```python
from build123d import *

# Parameters (mm, degrees)
F0_W     = 500
F0_H     = 340
F0_W_2   = 280
F0_W_3   = 150
F0_H_2   = 30
F1_DEPTH = 400


with BuildPart() as f1:
    # F0 (on Front) → F1 (new body)
    with BuildSketch(Plane.XZ):
        Polygon((698.162909, 183.718975), (-701.837091, 183.718975), (-701.837091, 143.844262), (-701.837091, 143.718975), (-701.837091, -216.281025), (-551.837091, -216.281025), (548.162909, -216.281025), (698.162909, -216.281025), (698.162909, -186.281025), (698.162909, 153.718975), align=None)
        with Locations((-421.837091, -16.281025)):
            Rectangle(F0_W, F0_H, mode=Mode.SUBTRACT)
        with Locations((-1.837091, -16.281025)):
            Rectangle(F0_W_2, F0_H, mode=Mode.SUBTRACT)
        with Locations((418.162909, -16.281025)):
            Rectangle(F0_W, F0_H, mode=Mode.SUBTRACT)
        with Locations((623.162909, -231.281025)):
            Rectangle(F0_W_3, F0_H_2)
        with Locations((418.162909, -16.281025)):
            Rectangle(F0_W, F0_H)
        with Locations((-626.837091, -231.281025)):
            Rectangle(F0_W_3, F0_H_2)
    extrude(amount=F1_DEPTH)


solid = f1.part
```
Model file for the job. Use its own axes, mm. A direction names the side the tool comes from. Give positions to 0.01 mm unless a question says otherwise; leave off trailing zeros. Loops run counter-clockwise (first coordinate to the right, second up) from the corner with the lowest first, then second, coordinate; pieces in that order, holes last. Notation, with made-up numbers: (61.5, 0.25) - (109.5, 0.25) arc R13 cw to (109.5, 21.25) - close; hole circle Ø4 at (-32.5, -26). An arc over 180 degrees is marked (long way). One line per item, written item: value. Start each with the question number.
1. Probe L1, parallel to X at y = -207, z = -79.5; L2, parallel to Z at x = 69, y = -340; L3, parallel to Z at x = 513, y = -81. List the from-to ranges inside material, lowest first. Write a range as from..to.
2. Slice it at D-D (x = 307). List the corners of the cut face in (y, z).
3. Pin check, flat tip, straight feed: pin 1 (6 mm diameter, centred on x = -35, y = -224.5, fed in from -Z). Stop position of the tip, or through.
4. Which spindle directions (+Z, -Z, +X, -X, +Y, -Y) get a long thin tool onto all of the face, cutting with end or side? Do faces 1 (the flat face through (-141.837, -197, -19)), 2 (the flat face through (144, 0, 20)), 3 (the flat face through (548.163, -197, -231)). Say none if no direction does.
5. Pull direction Z, two halves, no side cores. Call faces 4 (the flat face through (8, -197, 183.719)), 5 (the flat face through (-10, -197, -216.281)), 6 (the flat face through (-671.837, -197, -19)): pulls with the +Z half, pulls with the -Z half, needs draft (parallel to the pull), parting line crosses it, or undercut.
6. Slice it at C-C (y = -167). List the corners of the cut face in (x, z), plus the area to 3 significant figures.
7. Slice it at B-B (z = -47.5). List the corners of the cut face in (x, y).
8. Slice it at A-A (x = -477.5). List the corners of the cut face in (y, z), plus the area to 3 significant figures.
Solution:
1. L1: x = -701.84..-671.84, -171.84..-141.84, 138.16..698.16
1. L2: z = -216.28..-186.28, 153.72..183.72
1. L3: z = -216.28..183.72
2. outline: (-400, -216.28) - (0, -216.28) - (0, 183.72) - (-400, 183.72) - close
3. pin 1: stops at z = -216.28
4. face 1: +Y, -Y
4. face 2: +Z, -Z, +X, -X, +Y
4. face 3: -Z, +Y, -Y
5. face 4: pulls with the +Z half
5. face 5: pulls with the -Z half
5. face 6: undercut
6. outline: (-701.84, -246.28) - (-551.84, -246.28) - (-551.84, -216.28) - (548.16, -216.28) - (548.16, -246.28) - (698.16, -246.28) - (698.16, 183.72) - (-701.84, 183.72) - close; hole (-671.84, -186.28) - (-171.84, -186.28) - (-171.84, 153.72) - (-671.84, 153.72) - close; hole (-141.84, -186.28) - (138.16, -186.28) - (138.16, 153.72) - (-141.84, 153.72) - close
6. area: 304,000 mm^2
7. outline: (-701.84, -400) - (-671.84, -400) - (-671.84, 0) - (-701.84, 0) - close; (-171.84, -400) - (-141.84, -400) - (-141.84, 0) - (-171.84, 0) - close; (138.16, -400) - (698.16, -400) - (698.16, 0) - (138.16, 0) - close
8. outline: (-400, -216.28) - (0, -216.28) - (0, -186.28) - (-400, -186.28) - close; (-400, 153.72) - (0, 153.72) - (0, 183.72) - (-400, 183.72) - close
8. area: 24,000 mm^2
